CAD build for the part. Positions are in the model's coordinates, mm. Round coordinates to 2 decimals unless told otherwise and drop trailing zeros. Loops run counter-clockwise (first coordinate to the right, second up) from the corner with the lowest first, then second, coordinate; pieces in that order, holes last.
Autodesk Inventor part; units mm, degrees
ref_plane "YZ Plane" through (0, 0, 0) normal (1, 0, 0) x (0, 1, 0)
ref_plane "XZ Plane" through (0, 0, 0) normal (0, 1, 0) x (-1, 0, 0)
ref_plane "XY Plane" through (0, 0, 0) normal (0, 0, 1) x (1, 0, 0)
sketch "Sketch1" plane through (0, 0, 0) normal (0, 1, 0) x (-1, 0, 0)
  circle A0 centre (29.0135, 3.825) radius 1.05
  circle A1 centre (17.1265, 3.825) radius 1.05
  circle A2 centre (17.1265, 15.825) radius 1.05
  circle A3 centre (29.0135, 15.825) radius 1.05
  circle A4 centre (0, 9.96) radius 3.6
  circle A5 centre (45, 9.96) radius 3.6
  circle A6 centre (0, 16.96) radius 1.05
  circle A7 centre (-7, 9.96) radius 1.05
  circle A8 centre (0, 2.96) radius 1.05
  circle A9 centre (7, 9.96) radius 1.05
  circle A10 centre (45, 16.96) radius 1.05
  circle A11 centre (38, 9.96) radius 1.05
  circle A12 centre (45, 2.96) radius 1.05
  circle A13 centre (52, 9.96) radius 1.05
  arc A14 (45, 0) -> (45, 19.92) centre (45, 9.96) ccw
  line L0 (0, 19.92) -> (45, 19.92)
  arc A15 (0, 19.92) -> (0, 0) centre (0, 9.96) ccw
  line L1 (45, 0) -> (0, 0)
  point P0 (0, 0)
extrude "Extrusion1" add sketch "Sketch1" against normal blind 1.5
properties part number "axis_3_bottom_frame(bottom)" material "Aluminum 6061-AHC"
Item 1: Cut at C-C, the plane y = -1.2. State how many separate pieces and enclosed holes the cut face has, plus the area to 3 significant figures.
Answers follow:
separate pieces: 1
enclosed holes: 14
area: 1,090 mm2
Item 2: Cut at A-A, the plane x = -7. Give the cut face in (y, z), plus the area to 3 significant figures.
Answers follow:
outline: (-1.5, 0) - (0, 0) - (0, 8.91) - (-1.5, 8.91) - close; (-1.5, 11.01) - (0, 11.01) - (0, 19.92) - (-1.5, 19.92) - close
area: 26.7 mm2
Item 3: Two-plate mould, pull along X, no slides. Class faces 1 (the cylindrical face through (-17.611, -0.74, 2.893)), 2 (the flat face through (-23, -1, 0)), 3 (the cylindrical face through (-54.958, -0.74, 9.741)), 4 (the cylindrical face through (9.958, -0.74, 10.179)): released by +X, released by -X, zero draft, split by the parting line, or undercut.
Answers follow:
face 1: undercut
face 2: zero draft
face 3: released by -X
face 4: released by +X
Item 4: Probe line 1 (Z direction, x = -45, y = -1); line 2 (X direction, y = -0.6, z = 6.75); line 3 (X direction, y = -0.05, z = 3.25). List the from-to ranges inside material, lowest first.
Answers follow:
line 1: z = 0 to 1.91, 4.01 to 6.36, 13.56 to 15.91, 18.01 to 19.92
line 2: x = -54.43 to -46.63, -43.37 to -1.63, 1.63 to 9.43
line 3: x = -52.36 to -46.01, -43.99 to -29.89, -28.13 to -18.01, -16.25 to -1.01, 1.01 to 7.36
Item 5: Cut at B-B, the plane z = 9.96. Give the cut face in (x, y).
Answers follow:
outline: (-54.96, -1.5) - (-53.05, -1.5) - (-53.05, 0) - (-54.96, 0) - close; (-50.95, -1.5) - (-48.6, -1.5) - (-48.6, 0) - (-50.95, 0) - close; (-41.4, -1.5) - (-39.05, -1.5) - (-39.05, 0) - (-41.4, 0) - close; (-36.95, -1.5) - (-8.05, -1.5) - (-8.05, 0) - (-36.95, 0) - close; (-5.95, -1.5) - (-3.6, -1.5) - (-3.6, 0) - (-5.95, 0) - close; (3.6, -1.5) - (5.95, -1.5) - (5.95, 0) - (3.6, 0) - close; (8.05, -1.5) - (9.96, -1.5) - (9.96, 0) - (8.05, 0) - close
